Autodesk Inventor part; units mm, degrees
ref_plane "YZ Plane" through (0, 0, 0) normal (1, 0, 0) x (0, 1, 0)
ref_plane "XZ Plane" through (0, 0, 0) normal (0, 1, 0) x (-1, 0, 0)
ref_plane "XY Plane" through (0, 0, 0) normal (0, 0, 1) x (1, 0, 0)
sketch "Skizze1" plane through (0, 0, 0) normal (0, 0, 1) x (1, 0, 0)
  line L0 (-81, 132.5) -> (81, 132.5)
  line L1 (81, 132.5) -> (81, -132.5)
  line L2 (81, -132.5) -> (-81, -132.5)
  line L3 (-81, -132.5) -> (-81, 132.5)
  line L4 (-81, 132.5) -> (81, -132.5) construction
  line L5 (81, 132.5) -> (-81, -132.5) construction
  point P0 (0, 0)
  dimension "d0" = 162
  dimension "d1" = 265
extrude "Grobblech1" add sketch "Skizze1" along normal blind 2
fillet "Eckenrundung1" radius 10 4 edges at (-81, 132.5, 1) (81, 132.5, 1) (81, -132.5, 1) (-81, -132.5, 1)
sketch "Skizze2" plane through (0, 0, 2) normal (0, 0, 1) x (1, 0, 0)
  arc A0 (-81, -122.5) -> (-71, -132.5) centre (-71, -122.5) ccw
  line L0 (71, -132.5) -> (-71, -132.5)
  arc A1 (71, -132.5) -> (81, -122.5) centre (71, -122.5) ccw
  line L1 (81, 122.5) -> (81, -122.5)
  arc A2 (81, 122.5) -> (71, 132.5) centre (71, 122.5) ccw
  line L2 (-71, 132.5) -> (71, 132.5)
  arc A3 (-71, 132.5) -> (-81, 122.5) centre (-71, 122.5) ccw
  line L3 (-81, -122.5) -> (-81, 122.5)
  arc A4 (76, 122.5) -> (71, 127.5) centre (71, 122.5) ccw
  line L4 (76, 122.5) -> (76, -122.5)
  arc A5 (71, -127.5) -> (76, -122.5) centre (71, -122.5) ccw
  line L5 (71, -127.5) -> (-71, -127.5)
  arc A6 (-76, -122.5) -> (-71, -127.5) centre (-71, -122.5) ccw
  line L6 (-76, -122.5) -> (-76, 122.5)
  arc A7 (-71, 127.5) -> (-76, 122.5) centre (-71, 122.5) ccw
  line L7 (-71, 127.5) -> (71, 127.5)
  line L8 (-135.5785, 0) -> (231.9734, 0)
  line L9 (0, -191.312) -> (0, 205.8747)
  line L10 (-22.5, -117.5) -> (22.5, -117.5)
  line L11 (22.5, -117.5) -> (22.5, -122.5)
  line L12 (22.5, -122.5) -> (-22.5, -122.5)
  line L13 (-22.5, -122.5) -> (-22.5, -117.5)
  line L14 (30, -127.5) -> (30, -108.5)
  line L15 (30, -108.5) -> (-30, -108.5)
  line L16 (-30, -108.5) -> (-30, -127.5)
  line L17 (-53.5621, 127.5) -> (-20.4158, 127.5) construction
  point P0 (0, 0)
  dimension "d4" = 5
  dimension "d7" = 45
  dimension "d8" = 5
  dimension "d10" = 9
  dimension "d70" = 10
  dimension "d71" = 60
extrude "Ausklinkung1" cut sketch "Skizze2" against normal blind 2 contours L12 L13 L10 L9 | L9 L10 L11 L12
sketch "Skizze5" plane through (0, 0, 2) normal (0, 0, 1) x (1, 0, 0)
  line L0 (-22.5, -122.5) -> (-22.5, -117.5)
  line L1 (-22.5, -117.5) -> (22.5, -117.5)
  line L2 (22.5, -117.5) -> (22.5, -122.5)
  line L3 (22.5, -122.5) -> (-22.5, -122.5)
  arc A0 (-81, -122.5) -> (-71, -132.5) centre (-71, -122.5) ccw
  line L4 (71, -132.5) -> (-71, -132.5)
  arc A1 (71, -132.5) -> (81, -122.5) centre (71, -122.5) ccw
  line L5 (81, 122.5) -> (81, -122.5)
  arc A2 (81, 122.5) -> (71, 132.5) centre (71, 122.5) ccw
  line L6 (-71, 132.5) -> (71, 132.5)
  arc A3 (-71, 132.5) -> (-81, 122.5) centre (-71, 122.5) ccw
  line L7 (-81, -122.5) -> (-81, 122.5)
  arc A4 (-71, 127.5) -> (-76, 122.5) centre (-71, 122.5) ccw
  line L8 (-71, 127.5) -> (71, 127.5)
  arc A5 (76, 122.5) -> (71, 127.5) centre (71, 122.5) ccw
  line L9 (76, 122.5) -> (76, -122.5)
  arc A6 (71, -127.5) -> (76, -122.5) centre (71, -122.5) ccw
  line L10 (71, -127.5) -> (-71, -127.5)
  arc A7 (-76, -122.5) -> (-71, -127.5) centre (-71, -122.5) ccw
  line L11 (-76, -122.5) -> (-76, 122.5)
  line L12 (26.5, -108.5) -> (-26.5, -108.5)
  line L13 (-31.5, -113.5) -> (-31.5, -132.5)
  line L14 (-31.5, -132.5) -> (31.5, -132.5)
  line L15 (31.5, -132.5) -> (31.5, -113.5)
  line L16 (-81, -122.5) -> (-81, 122.5)
  line L17 (31.5, -127.5) -> (-31.5, -127.5)
  line L18 (-31.5, -127.5) -> (-31.5, -113.5)
  line L19 (-26.5, -108.5) -> (26.5, -108.5)
  line L20 (31.5, -113.5) -> (31.5, -127.5)
  arc A8 (-26.5, -108.5) -> (-31.5, -113.5) centre (-26.5, -113.5) ccw
  arc A9 (31.5, -113.5) -> (26.5, -108.5) centre (26.5, -113.5) ccw
  line L21 (71, -132.5) -> (-71, -132.5)
  point P0 (0, 0)
  point P1 (31.5, -108.5)
  dimension "d37" = 5
  dimension "d38" = 9
  dimension "d41" = 5
extrude "Ausklinkung2" cut sketch "Skizze5" against normal blind 2 contours L10 A7 L11 A4 L8 A5 L9 A6 L15 A9 L12 A8 L13
equation "\"d17\" = Stärke"
equation "\"d39\" = Stärke"
equation "\"d2\" = Stärke"
equation "\"Biegeradius\" = Stärke"
equation "\"BreiteBiegungsfreistellung\" = Stärke"
equation "\"TiefeBiegungsfreistellung\" = 0.5 * Stärke"
equation "\"GrößeEckenfreistellung\" = 4 * Stärke"
equation "\"MinimalRest\" = 2 * Stärke"
equation "\"Übergangsradius\" = Biegeradius"
equation "\"JacobiRadiusGröße\" = Biegeradius"
equation "\"Abstandsgröße\" = Stärke"
properties part number "Rost_Basis"
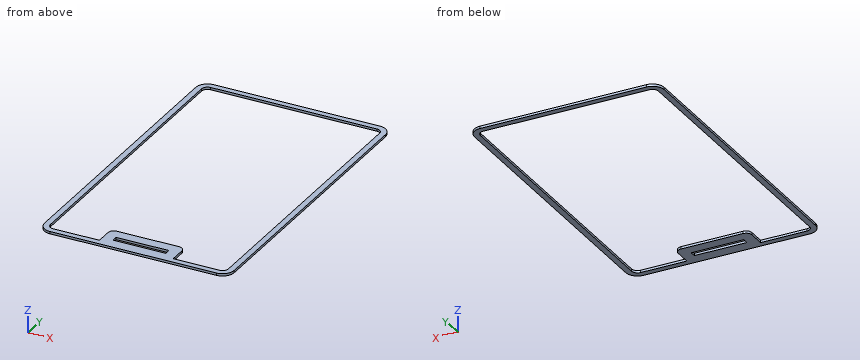
Could you check a few things on this model? Use its own coordinates, in mm. Give positions to 0.01 mm unless a question says otherwise; leave off trailing zeros. Order: outer loops, then holes, each group sorted by start corner. A loop starts at its lowest first (then second) coordinate and runs counter-clockwise, first axis right, second up.
Q1. Suppose I cut it at B-B, the plane z = 0.7. Write out the boundary of the cut face in (x, y), and give its area (3 significant figures).
Q2. Suppose I cut it at D-D, the plane y = -91. Write out the boundary of the cut face in (x, z).
Q3. Suppose I cut it at C-C, the plane x = 16. Write out the boundary of the cut face in (y, z).
Q4. Suppose I cut it at A-A, the plane x = 60.5. Write out the boundary of the cut face in (y, z), and give its area (3 significant figures).
Q5. If I drill on line 1 along Y through (x, z) = (19, 1.9); line 2 along X through (y, z) = (-58.5, 0.7); line 3 along Y through (x, z) = (-63.5, 1.1), over which ranges is the centre line in solid material (lowest first)?
Solution:
1. outline: (-81, -122.5) arc R10 ccw to (-71, -132.5) - (71, -132.5) arc R10 ccw to (81, -122.5) - (81, 122.5) arc R10 ccw to (71, 132.5) - (-71, 132.5) arc R10 ccw to (-81, 122.5) - close; hole (-76, -122.5) arc R5 ccw to (-71, -127.5) - (-31.5, -127.5) - (-31.5, -113.5) arc R5 cw to (-26.5, -108.5) - (26.5, -108.5) arc R5 cw to (31.5, -113.5) - (31.5, -127.5) - (71, -127.5) arc R5 ccw to (76, -122.5) - (76, 122.5) arc R5 ccw to (71, 127.5) - (-71, 127.5) arc R5 ccw to (-76, 122.5) - close; hole (-22.5, -122.5) - (22.5, -122.5) - (22.5, -117.5) - (-22.5, -117.5) - close
1. area: 5,070 mm2
2. outline: (-81, 0) - (-76, 0) - (-76, 2) - (-81, 2) - close; (76, 0) - (81, 0) - (81, 2) - (76, 2) - close
3. outline: (-132.5, 0) - (-122.5, 0) - (-122.5, 2) - (-132.5, 2) - close; (-117.5, 0) - (-108.5, 0) - (-108.5, 2) - (-117.5, 2) - close; (127.5, 0) - (132.5, 0) - (132.5, 2) - (127.5, 2) - close
4. outline: (-132.5, 0) - (-127.5, 0) - (-127.5, 2) - (-132.5, 2) - close; (127.5, 0) - (132.5, 0) - (132.5, 2) - (127.5, 2) - close
4. area: 20.0 mm2
5. line 1: y = -132.5 to -122.5, -117.5 to -108.5, 127.5 to 132.5
5. line 2: x = -81 to -76, 76 to 81
5. line 3: y = -132.5 to -127.5, 127.5 to 132.5
